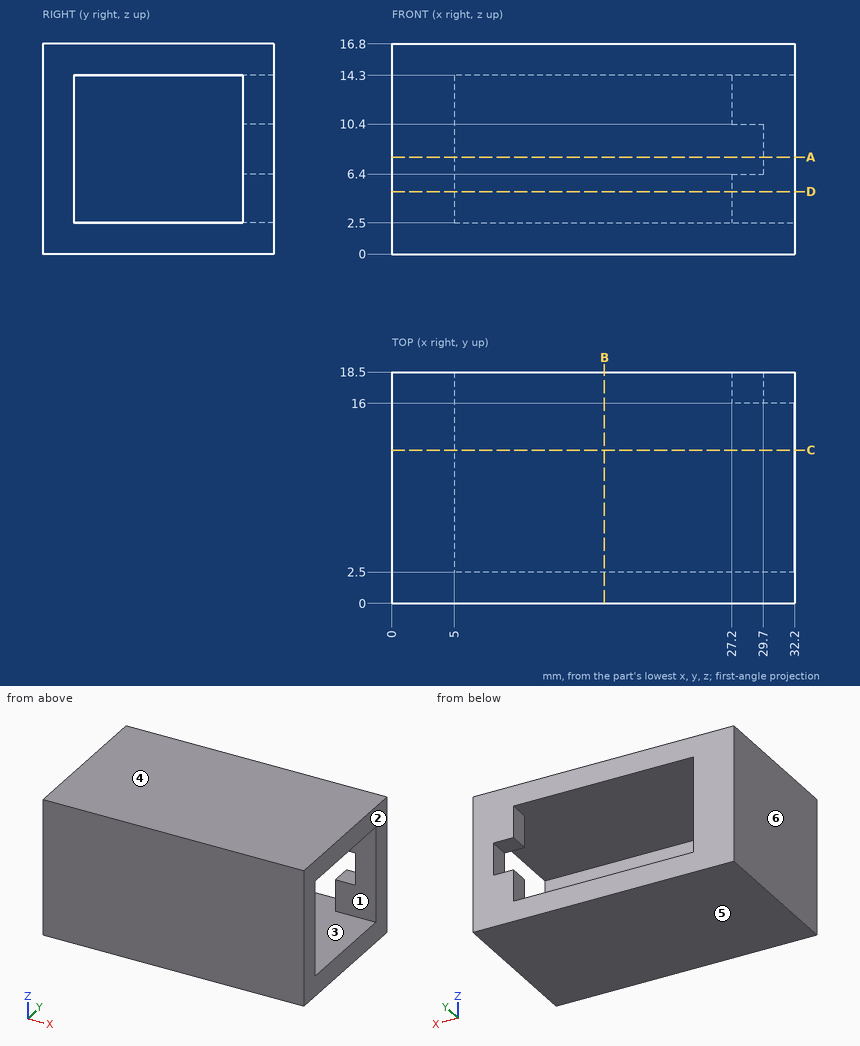
Study the drawing (mm; zero at the part's minimum x, y, z) and answer. A direction names the side the tool comes from. Give positions to 0.01 mm unless a question says otherwise; leave off trailing zeros. Order: outer loops, then holes, each group sorted by start corner. A loop starts at its lowest first (then second) coordinate and runs counter-clockwise, first axis right, second up. Notation, with made-up numbers: M 78.5,-5.5 L 132.5,-5.5 A15 cw 132.5,22.5 Z; hole C 63.25,77 d11. An arc over 180 degrees is marked long. Put each result on its own line as item: value. Start each with the question number.
Item 1: A flat-ended cylindrical pin translates along its axis: P1, Ø2, axis at y = 16.5, z = 9, coming from the -X side. Find the tip coordinate at first contact, or state that the pin passes through.
Item 2: The part is cut by section B-B, the plane x = 17. Determine the outline of the cut face in (y, z).
Item 3: The part is cut by section A-A, the plane z = 7.75. Determine the outline of the cut face in (x, y), and give its area (3 significant figures).
Item 4: The part is cut by section C-C, the plane y = 12.25. Determine the outline of the cut face in (x, z).
Item 5: The part is cut by section D-D, the plane z = 5. Determine the outline of the cut face in (x, y).
Item 6: Find the intervals of material crossed by line 1 along Z through (x, y) = (12, 15.5); line 2 along Y through (x, z) = (30, 3.5); line 3 along X through (y, z) = (17, 4.5), in increasing order.
Item 7: Which of the six approach directions +Z, -Z, +X, -X, +Y, -Y give full straight-line access (tool end or side, diameter ignored) to the marked faces 1 and 2?
Item 8: For a pull along Z with two mould halves and no side action, classify the marked faces 3, 4, 5 and 6 as +Z half, -Z half, draft (parallel to the pull), parting line (faces both ways), or undercut.
Answer key:
1. P1: stops at x = 0
2. outline: M 0,0 L 18.5,0 L 18.5,2.5 L 2.5,2.5 L 2.5,14.3 L 18.5,14.3 L 18.5,16.8 L 0,16.8 Z
3. outline: M 0,0 L 32.2,0 L 32.2,2.5 L 5,2.5 L 5,18.5 L 0,18.5 Z; M 29.7,16 L 32.2,16 L 32.2,18.5 L 29.7,18.5 Z
3. area: 167 mm²
4. outline: M 0,0 L 32.2,0 L 32.2,2.5 L 5,2.5 L 5,14.3 L 32.2,14.3 L 32.2,16.8 L 0,16.8 Z
5. outline: M 0,0 L 32.2,0 L 32.2,2.5 L 5,2.5 L 5,18.5 L 0,18.5 Z; M 27.2,16 L 32.2,16 L 32.2,18.5 L 27.2,18.5 Z
6. line 1: z = 0 to 2.5, 14.3 to 16.8
6. line 2: y = 0 to 2.5, 16 to 18.5
6. line 3: x = 0 to 5, 27.2 to 32.2
7. face 1: +X
7. face 2: +Z, -Z, +X, +Y, -Y
8. face 3: undercut
8. face 4: +Z half
8. face 5: -Z half
8. face 6: draft
